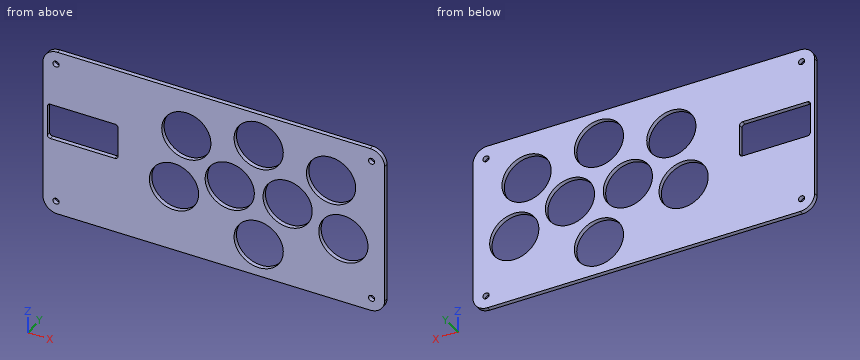
from build123d import *

# Parameters (mm, degrees)
SKETCH1_W           = 236
SKETCH1_H           = 118.5
SKETCH1_W_2         = 48.8
SKETCH1_H_2         = 25.1
SKETCH1_R           = 17
SKETCH1_R_2         = 2.125
BOSS_EXTRUDE1_DEPTH = 3
FILLET1_R           = 10
FILLET2_R           = 2


with BuildPart() as part:
    # Sketch1 → Boss-Extrude1 (new body)
    with BuildSketch(Plane(origin=(0, 0, 0), x_dir=(1, 0, 0), z_dir=(0, 1, 0))):
        with Locations((64.335496373, 41.57608502)):
            Rectangle(SKETCH1_W, SKETCH1_H)
        with Locations((-26.264503627, 34.57608502)):
            Rectangle(SKETCH1_W_2, SKETCH1_H_2, mode=Mode.SUBTRACT)
        with Locations(Location((75.335496373, 41.57608502, 0), (0, 0, 270))):
            Circle(SKETCH1_R, mode=Mode.SUBTRACT)
        with Locations(Location((115.335496373, 41.57608502, 0), (0, 0, 270))):
            Circle(SKETCH1_R, mode=Mode.SUBTRACT)
        with Locations(Location((153.835496373, 54.57608502, 0), (0, 0, 270))):
            Circle(SKETCH1_R, mode=Mode.SUBTRACT)
        with Locations(Location((95.335496373, 77.82608502, 0), (0, 0, 270))):
            Circle(SKETCH1_R, mode=Mode.SUBTRACT)
        with Locations(Location((173.335496373, 91.82608502, 0), (0, 0, 270))):
            Circle(SKETCH1_R_2, mode=Mode.SUBTRACT)
        with Locations(Location((-44.664503627, -8.67391498, 0), (0, 0, 270))):
            Circle(SKETCH1_R_2, mode=Mode.SUBTRACT)
        with Locations(Location((45.335496373, 14.57608502, 0), (0, 0, 270))):
            Circle(SKETCH1_R, mode=Mode.SUBTRACT)
        with Locations(Location((95.335496373, 5.32608502, 0), (0, 0, 270))):
            Circle(SKETCH1_R, mode=Mode.SUBTRACT)
        with Locations(Location((173.335496373, -8.67391498, 0), (0, 0, 270))):
            Circle(SKETCH1_R_2, mode=Mode.SUBTRACT)
        with Locations(Location((145.335496373, 14.57608502, 0), (0, 0, 270))):
            Circle(SKETCH1_R, mode=Mode.SUBTRACT)
        with Locations(Location((36.835496373, 54.57608502, 0), (0, 0, 270))):
            Circle(SKETCH1_R, mode=Mode.SUBTRACT)
        with Locations(Location((-44.664503627, 91.82608502, 0), (0, 0, 270))):
            Circle(SKETCH1_R_2, mode=Mode.SUBTRACT)
    extrude(amount=BOSS_EXTRUDE1_DEPTH)

    # Fillet1
    fillet1_edges = [part.edges().sort_by_distance(p)[0] for p in [
        (182.335496373, 1.5, -100.82608502),
        (182.335496373, 1.5, 17.67391498),
        (-53.664503627, 1.5, 17.67391498),
        (-53.664503627, 1.5, -100.82608502),
    ]]
    fillet(fillet1_edges, radius=FILLET1_R)

    # Fillet2
    fillet2_edges = [part.edges().sort_by_distance(p)[0] for p in [
        (-50.664503627, 1.5, -22.02608502),
        (-1.864503627, 1.5, -22.02608502),
        (-1.864503627, 1.5, -47.12608502),
        (-50.664503627, 1.5, -47.12608502),
    ]]
    fillet(fillet2_edges, radius=FILLET2_R)


solid = part.part
Model file for the job. Use its own axes, mm. Give positions to 0.01 mm unless a question says otherwise; leave off trailing zeros. Write each loop counter-clockwise with the first axis right and the second up, starting at its lowest first coordinate (ties: lowest second). Pieces come first, ordered by that corner, then holes. Notation, with made-up numbers: (78, 77) -> (91, 77) arc R20 ccw to (91, 82) -> close; hole circle Ø9 at (3, 3.25). An arc over 180 degrees is marked (long way). Write item = value, one per line.
(1) Slice it at B-B, the plane x = 90. Give the cut face in (y, z).
Determined:
outline = (0, -100.83) -> (3, -100.83) -> (3, -93.97) -> (0, -93.97) -> close; (0, -61.69) -> (3, -61.69) -> (3, -50.18) -> (0, -50.18) -> close; (0, -32.98) -> (3, -32.98) -> (3, -21.47) -> (0, -21.47) -> close; (0, 10.81) -> (3, 10.81) -> (3, 17.67) -> (0, 17.67) -> close
(2) Probe line 1 along Z through (x, y) = (-26.5, 0.4); line 2 along X through (y, z) = (2.45, -77.5); line 3 along Z through (x, y) = (104.5, 1.55). List the from-to ranges inside material, lowest first.
Determined:
line_1 = -100.83 to -47.13, -22.03 to 17.67
line_2 = -53.66 to 78.34, 112.33 to 182.34
line_3 = -100.83 to -92.14, -63.51 to -54.68, -28.48 to -19.64, 8.99 to 17.67
(3) Flat gauge pins, fed straight in: P1, Ø5, axis at x = -44.66, z = -91.83, coming from the +Y side; P2, Ø4, axis at x = 173.34, z = -91.83, coming from the -Y side. Where does each tip first touch, or does it go through?
Determined:
P1 = 3
P2 = through
(4) Slice it at A-A, the plane z = -4. Give the cut face in (x, y), then the cut area to 3 significant figures.
Determined:
outline = (-53.66, 0) -> (32.03, 0) -> (32.03, 3) -> (-53.66, 3) -> close; (58.65, 0) -> (78.39, 0) -> (78.39, 3) -> (58.65, 3) -> close; (112.28, 0) -> (132.03, 0) -> (132.03, 3) -> (112.28, 3) -> close; (158.65, 0) -> (182.34, 0) -> (182.34, 3) -> (158.65, 3) -> close
area = 447 mm2
(5) Slice it at C-C, the plane x = 31.5. Give the cut face in (y, z), then the cut area to 3 significant figures.
Determined:
outline = (0, -100.83) -> (3, -100.83) -> (3, -70.72) -> (0, -70.72) -> close; (0, -38.44) -> (3, -38.44) -> (3, -24.45) -> (0, -24.45) -> close; (0, -4.7) -> (3, -4.7) -> (3, 17.67) -> (0, 17.67) -> close
area = 199 mm2
(6) Slice it at D-D, the plane y = 0.75. Give the number of separate pieces and of enclosed holes in the cut face, then the cut area to 3 significant figures.
Determined:
separate_pieces = 1
enclosed_holes = 13
area = 19,300 mm2
